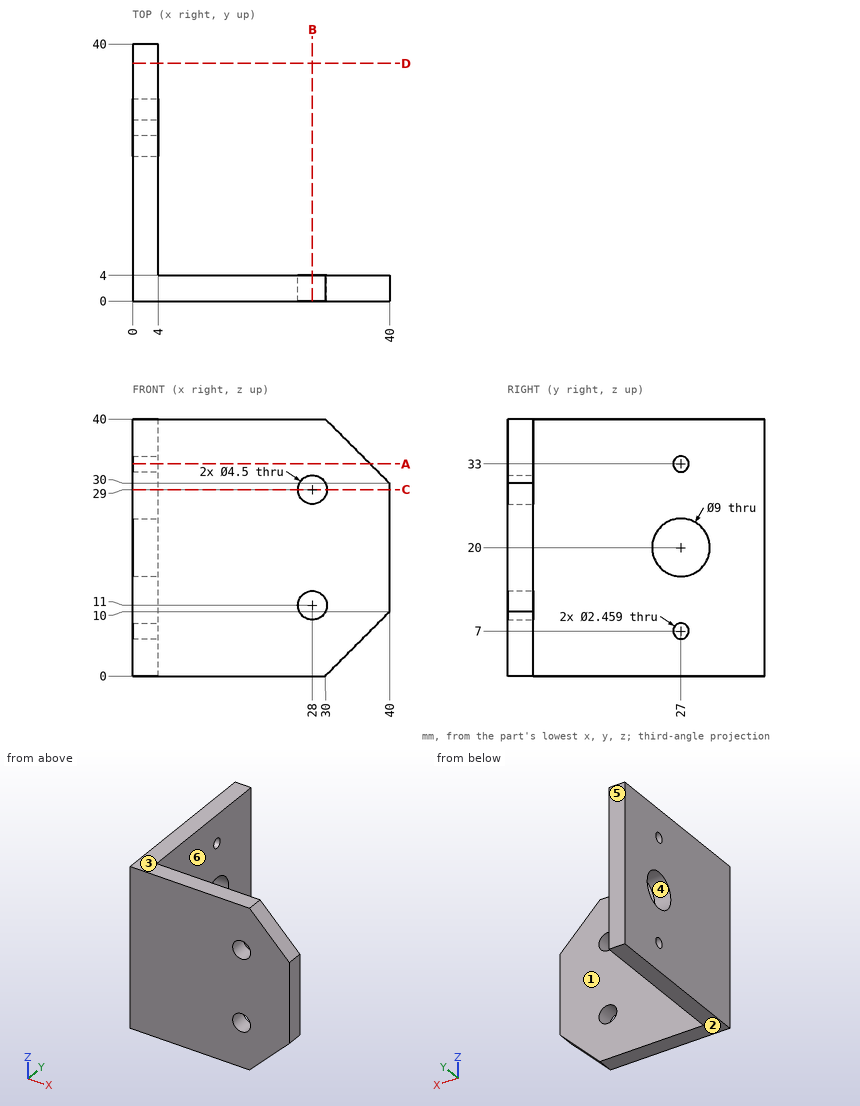
The figure shows three views and two pictorial views of one solid part (mm, origin at its lowest corner). Answer the questions. A direction names the side the tool comes from. Give positions to 0.01 mm unless a question says otherwise; leave off trailing zeros. Order: outer loops, then holes, each group sorted by start corner. A loop starts at its lowest first (then second) coordinate and runs counter-clockwise, first axis right, second up. Notation, with made-up numbers: (-18.75, 64) -> (7.25, 64) arc R17 cw to (7.25, 87) -> close; hole circle Ø1 at (-39.5, 18). An arc over 180 degrees is marked (long way). One line per item, written item: value.
1) Find section A-A, the plane z = 33. Determine the outline of the cut face in (x, y).
Reported:
outline: (0, 0) -> (37, 0) -> (37, 4) -> (4, 4) -> (4, 25.77) -> (0, 25.77) -> close; (0, 28.23) -> (4, 28.23) -> (4, 40) -> (0, 40) -> close
2) Find section B-B, the plane x = 28. Determine the outline of the cut face in (y, z), plus the area to 3 significant figures.
Reported:
outline: (0, 0) -> (4, 0) -> (4, 8.75) -> (0, 8.75) -> close; (0, 13.25) -> (4, 13.25) -> (4, 26.75) -> (0, 26.75) -> close; (0, 31.25) -> (4, 31.25) -> (4, 40) -> (0, 40) -> close
area: 124 mm^2
3) Find the intervals of material crossed by line 1 (Z direction, x = 1, y = 27); line 2 (Z direction, x = 28, y = 1); line 3 (X direction, y = 2.85, z = 29), in increasing order.
Reported:
line 1: z = 0 to 5.77, 8.23 to 15.5, 24.5 to 31.77, 34.23 to 40
line 2: z = 0 to 8.75, 13.25 to 26.75, 31.25 to 40
line 3: x = 0 to 25.75, 30.25 to 40
4) Find section D-D, the plane y = 37. Determine the outline of the cut face in (x, z).
Reported:
outline: (0, 0) -> (4, 0) -> (4, 40) -> (0, 40) -> close
5) Find section C-C, the plane z = 29. Determine the outline of the cut face in (x, y), plus the area to 3 significant figures.
Reported:
outline: (0, 0) -> (25.75, 0) -> (25.75, 4) -> (4, 4) -> (4, 40) -> (0, 40) -> close; (30.25, 0) -> (40, 0) -> (40, 4) -> (30.25, 4) -> close
area: 286 mm^2
6) A tool of negligible diameter and unlimited length cuts with its end or side. For the marked faces 5 and 6, from which of +Z, -Z, +X, -X, +Y, -Y can it reach the whole face along a straight path? Write none if from no direction.
Reported:
face 5: +Z, -Z, +X, -X, +Y
face 6: +Z, -Z, +X, +Y
7) Flat-ended cylindrical pins translate along their axes: P1, Ø2, axis at y = 26.5, z = 34.5, coming from the +X side; P2, Ø1.5, axis at x = 6, z = 25.5, coming from the +Y side. Find the tip coordinate at first contact, or state that the pin passes through.
Reported:
P1: stops at x = 4
P2: stops at y = 4
8) Determine the mould class of the marked faces 1, 2, 3 and 4 for opening direction Z: pulls with the +Z half, pulls with the -Z half, needs draft (parallel to the pull), parting line crosses it, or undercut.
Reported:
face 1: needs draft
face 2: pulls with the -Z half
face 3: pulls with the +Z half
face 4: undercut
